from build123d import *

# Parameters (mm, degrees)
BOSS_EXTRUDE1_DEPTH = 3.175
SKETCH2_W           = 38
SKETCH2_H           = 15
CUT_EXTRUDE1_DEPTH  = 4.175
FILLET1_R           = 4
FILLET2_R           = 10
SKETCH3_R           = 2.75
CUT_EXTRUDE2_DEPTH  = 4.175


with BuildPart() as part:
    # Sketch1 → Boss-Extrude1 (new body)
    with BuildSketch(Plane.XY):
        Polygon((32.5, 120), (-32.5, 120), (-32.5, 95), (0, 0), (32.5, 95), align=None)
    extrude(amount=BOSS_EXTRUDE1_DEPTH)

    # Sketch2 → Cut-Extrude1 (cut, through all)
    with BuildSketch(Plane.XY.offset(3.175)):
        with Locations((0, 112.5)):
            Rectangle(SKETCH2_W, SKETCH2_H)
        with BuildLine():
            Line((-26, 117.6), (-24, 117.6))
            ThreePointArc((-24, 117.6), (-21.4, 115), (-24, 112.4))
            Line((-24, 112.4), (-26, 112.4))
            ThreePointArc((-26, 112.4), (-28.6, 115), (-26, 117.6))
        make_face()
        with BuildLine():
            Line((26, 117.6), (24, 117.6))
            ThreePointArc((24, 117.6), (21.4, 115), (24, 112.4))
            Line((24, 112.4), (26, 112.4))
            ThreePointArc((26, 112.4), (28.6, 115), (26, 117.6))
        make_face()
    extrude(amount=-CUT_EXTRUDE1_DEPTH, mode=Mode.SUBTRACT)

    # Fillet1
    fillet1_edges = [part.edges().sort_by_distance(p)[0] for p in [
        (-19, 105, 1.5875),
        (-19, 120, 1.5875),
        (19, 120, 1.5875),
        (19, 105, 1.5875),
        (-32.5, 95, 1.5875),
        (-32.5, 120, 1.5875),
        (32.5, 120, 1.5875),
        (32.5, 95, 1.5875),
    ]]
    fillet(fillet1_edges, radius=FILLET1_R)

    # Fillet2
    fillet2_edges = [part.edges().sort_by_distance(p)[0] for p in [
        (0, 0, 1.5875),
    ]]
    fillet(fillet2_edges, radius=FILLET2_R)

    # Sketch3 → Cut-Extrude2 (cut, through all)
    with BuildSketch(Plane.XY.offset(3.175)):
        with Locations((0, 30.893977889)):
            Circle(SKETCH3_R)
    extrude(amount=-CUT_EXTRUDE2_DEPTH, mode=Mode.SUBTRACT)


solid = part.part
Geometry check sheet. Reference: the model listing, model coordinates, mm. A direction names the side the tool comes from. Give positions to 0.01 mm unless a question says otherwise; leave off trailing zeros. Write each loop counter-clockwise with the first axis right and the second up, starting at its lowest first coordinate (ties: lowest second). Pieces come first, ordered by that corner, then holes. Notation, with made-up numbers: M 59.5,17.5 L 79.5,17.5 A24 cw 79.5,55.5 Z; hole C -21.5,34.5 d10. An arc over 180 degrees is marked long. Answer as CSV lines item,"result". Start each with the question number.
Q1. Section check C-C, the plane z = 0.8. Record the cut outline in (x, y).
Q2. Section check B-B, the plane x = 0. Record the cut outline in (y, z) (3 decimals), then the cut area to 3 significant figures.
Q3. Tool access check on faces 1 (the face through (19, 112, 2)), 2 (the face through (25, 117.6, 2)), 3 (the face through (-21.033, 61.481, 1.565)). Record the directions out of +Z, -Z, +X, -X, +Y, -Y that give a thin tool (end or side, any length) a straight path to the whole face; none if there is none.
Q4. Release check for a two-part mould opening along X. For faces 4 (the face through (28.6, 114.9, 1.6)), 5 (the face through (20.713, 60.547, 1.565)), 6 (the face through (-31.359, 118.797, 1.61)), 7 (the face through (0.174, 20.895, 1.61)) record: pulls with the +X half, pulls with the -X half, needs draft (parallel to the pull), parting line crosses it, or undercut.
Q5. Go/stop test with flat-tipped pins: pin 1 (1.5 mm diameter, centred on y = 48, z = 0.5, fed in from +X); pin 2 (1 mm diameter, centred on x = -1, z = 1, fed in from +Y). Record where each tip stops, or that it passes through.
Q6. Material ranges on L1, parallel to Y at x = 0, z = 2.4; L2, parallel to X at y = 112, z = 1.4; L3, parallel to X at y = 115.5, z = 2.7, recorded low to high.
Q7. Section check A-A, the plane y = 115. Record the cut outline in (x, z) (3 decimals).
Q8. Section check D-D, the plane x = 6.5. Record the cut outline in (y, z) (3 decimals), then the cut area to 3 significant figures.
Geometry says:
1,outline,"M -32.5,95.67 A4 ccw -32.28,94.37 L -9.46,27.66 A10 ccw 9.46,27.66 L 32.28,94.37 A4 ccw 32.5,95.67 L 32.5,116 A4 ccw 28.5,120 L 23,120 A4 ccw 19,116 L 19,109 A4 cw 15,105 L -15,105 A4 cw -19,109 L -19,116 A4 ccw -23,120 L -28.5,120 A4 ccw -32.5,116 Z; hole M -26,112.4 L -24,112.4 A2.6 ccw -24,117.6 L -26,117.6 A2.6 ccw Z; hole C 0,30.89 d5.5; hole M 24,112.4 L 26,112.4 A2.6 ccw 26,117.6 L 24,117.6 A2.6 ccw Z"
2,outline,"M 20.894,0 L 28.144,0 L 28.144,3.175 L 20.894,3.175 Z; M 33.644,0 L 105,0 L 105,3.175 L 33.644,3.175 Z"
2,area,"250 mm^2"
3,face 1,"+Z, -Z, +Y"
3,face 2,"+Z, -Z"
3,face 3,"+Z, -Z, -X, -Y"
4,face 4,"undercut"
4,face 5,"pulls with the +X half"
4,face 6,"pulls with the -X half"
4,face 7,"parting line crosses it"
5,pin 1,"x = 16.68"
5,pin 2,"y = 105"
6,L1,"20.89 to 28.14, 33.64 to 105"
6,L2,"-32.5 to -19, 19 to 32.5"
6,L3,"-32.5 to -28.55, -21.45 to -19, 19 to 21.45, 28.55 to 32.5"
7,outline,"M -32.5,0 L -28.6,0 L -28.6,3.175 L -32.5,3.175 Z; M -21.4,0 L -19,0 L -19,3.175 L -21.4,3.175 Z; M 19,0 L 21.4,0 L 21.4,3.175 L 19,3.175 Z; M 28.6,0 L 32.5,0 L 32.5,3.175 L 28.6,3.175 Z"
8,outline,"M 23.295,0 L 105,0 L 105,3.175 L 23.295,3.175 Z"
8,area,"259 mm^2"
